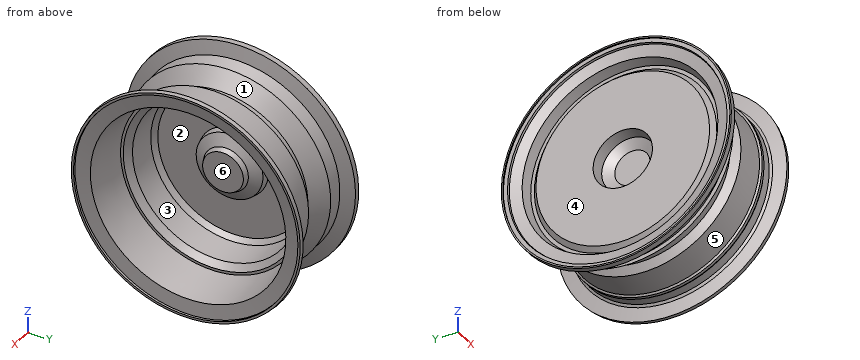
from build123d import *


with BuildPart() as f1:
    # F0 (on Front) → F1 (revolve)
    with BuildSketch(Plane.XZ):
        Polygon((5.101309, 70.075877), (0, 70.075877), (0, 68.68496), (1.546612, 69.017775), (1.546612, 65.19179), (3.493164, 64.654812), (5.775328, 54.049462), (14.635496, 51.230315), (14.635496, 47.836304), (10.16725, 43.687928), (10.16725, -9.660219), (20.394862, -11.620327), (25.411999, -20.876987), (25.411999, -37.358359), (32.686792, -37.358359), (32.686792, -18.305814), (28.057085, -16.390074), (22.309862, -6.172789), (16.10519, -4.842204), (16.10519, 33.313304), (20.394862, 37.377201), (45.050226, 39.85405), (50.47816, 45.281984), (50.47816, 47.836304), (87.826721, 53.909241), (89.407131, 67.406461), (91.588087, 67.406461), (91.588087, 69.501564), (87.826721, 70.075877), (85.940949, 57.725336), (84.473111, 55.494221), (77.600193, 54.583474), (76.215856, 55.494221), (73.410715, 55.494221), (72.228983, 53.697988), (47.168646, 51.145699), (42.422369, 43.931354), (35.967432, 43.931354), (23.358624, 57.725336), (23.358624, 53.697988), (8.860168, 57.725336), align=None)
    revolve(axis=Axis((29.049396, 0, -37.358359), (-1, 0, 0)))


solid = f1.part
CAD build for the part. Positions are in the model's coordinates, mm. Face numbers are marked on the shaded views. A direction names the side the tool comes from. Coordinates: 2 decimals unless noted, no trailing zeros. Write item = value, one per line. Start each with the question number.
Q1. Flat gauge pins, fed straight in: pin 1 Ø10 at (x, z) = (36, -97.5) entering from -Y; pin 2 Ø1.5 at (y, z) = (-79.5, 10) entering from -X; pin 3 Ø8 at (x, y) = (75.5, -55.5) entering from -Z. Where does each tip first touch, or does it go through?
Q2. Drill centre lines: L1, parallel to Z at x = 35, y = 51; L2, parallel to Z at x = 9, y = -82; L3, parallel to X at y = -21, z = -95.5. Where is each one in solid material? Low to high.
Q3. Pull direction Y, two halves, no side cores. Call the marked faces 1, 2 and 3: pulls with the +Y half, pulls with the -Y half, needs draft (parallel to the pull), parting line crosses it, or undercut.
Q4. Which spindle directions (+Z, -Z, +X, -X, +Y, -Y) get a long thin tool onto all of the face, cutting with end or side? Do the marked faces 4, 5 and 6. Say none if no direction does.
Computed:
q1.pin_1 = -63.81
q1.pin_2 = 5.37
q1.pin_3 = -114.62
q2.L1 = -102.01 to -93.98, 19.26 to 27.3
q2.L2 = -85.42 to -75.37, 0.65 to 10.7
q2.L3 = 10.17 to 16.11
q3.face_1 = parting line crosses it
q3.face_2 = undercut
q3.face_3 = undercut
q4.face_4 = -X
q4.face_5 = none
q4.face_6 = +X
